For this review, take the finished solid that the model builds, in its own axes (mm). Face numbers are marked on the shaded views. A direction names the side the tool comes from. Give positions to 0.01 mm unless a question says otherwise; leave off trailing zeros. Write each loop counter-clockwise with the first axis right and the second up, starting at its lowest first coordinate (ties: lowest second). Pieces come first, ordered by that corner, then holes.
1) Wall thickness on line 1 along X through (y, z) = (-14.5, 2); line 2 along Z through (x, y) = (-6.5, -34); line 3 along X through (y, z) = (-19.25, 2.3): over which ranges is each line inside the solid? List them lowest first.
2) We need section A-A on x = 0. Give the boundary of the cut face in (y, z), and give its area (3 significant figures).
3) We need section B-B on x = 9.5. Give the boundary of the cut face in (y, z), and give its area (3 significant figures).
4) We need section C-C on x = -5.5. Give the boundary of the cut face in (y, z).
5) Machinability: for the marked faces 4 and 5, which of the approach directions +Z, -Z, +X, -X, +Y, -Y give a long, thin tool a straight path to every point of the face, cutting with its end or side? Answer none if there is none.
6) For P1, Ø2, axis at x = -5, y = -18.5, coming from the -Z side; P2, Ø1.5, axis at x = -10.5, z = -3, coming from the -Y side; P3, Ø1.5, axis at x = 8, z = -1.5, coming from the -Y side, all flat-tipped, find the tip position at first contact; note any pin that passes through.
7) Draft analysis for pull direction X (two halves, no side actions). For the marked faces 1, 2 and 3, state which applies: pulls with the +X half, pulls with the -X half, needs draft (parallel to the pull), parting line crosses it, or undercut.
from build123d import *

# Parameters (mm, degrees)
EXTRUDE_1_DEPTH     = 4
EXTRUDE_START       = -10
EXTRUDE_2_DEPTH     = 10
EXTRUDE_3_DEPTH     = 10
CUT_EXTRUDE_1_DEPTH = 80.60065996608486
FILLET_1_R          = 2


with BuildPart() as part:
    # 草图1 → 凸台-拉伸1 (new body)
    with BuildSketch(Plane.XY):
        with BuildLine():
            ThreePointArc((10.284601754984639, -12.256711089903641), (5.472322293210865, -15.035081932574474), (3.3812e-13, -16))
            Line((0, -16), (0, -17.75))
            ThreePointArc((-1.91e-15, -17.75), (1.0606601717798214, -18.189339828220177), (1.5000000000000009, -19.25))
            ThreePointArc((1.5000000000000009, -19.25), (1.0606601717798207, -20.310660171779823), (-2.94e-15, -20.75))
            Line((0, -20.75), (0, -23.100000000000005))
            ThreePointArc((-4.24e-15, -23.100000000000005), (7.900665310822955, -21.706899540154488), (14.848393783759075, -17.695626636048384))
            Line((14.848393783759088, -17.695626636048377), (10.28460175498465, -12.256711089903638))
        make_face()
        with BuildLine():
            Line((0, -17.75), (0, -16))
            ThreePointArc((3.3812e-13, -16), (-5.472322293210549, -15.035081932574588), (-10.284601754984644, -12.256711089903638))
            Line((-10.284601754984646, -12.25671108990364), (-14.848393783759084, -17.69562663604838))
            ThreePointArc((-14.848393783759082, -17.69562663604838), (-7.900665310822965, -21.706899540154485), (-4.24e-15, -23.100000000000005))
            Line((0, -23.100000000000005), (0, -20.75))
            ThreePointArc((-2.94e-15, -20.75), (-1.5000000000000009, -19.25), (-2.24e-15, -17.75))
        make_face()
    extrude(amount=EXTRUDE_1_DEPTH)

    # 草图3 → 凸台-拉伸2 (add)
    with BuildSketch(Plane.XY.offset(4).offset(EXTRUDE_START)):
        with BuildLine():
            ThreePointArc((14.848393783759091, -17.695626636048377), (3.55e-15, -23.100000000000012), (-14.848393783759086, -17.69562663604838))
            Line((-14.848393783759084, -17.69562663604838), (-17.676659266379858, -21.066222185771874))
            ThreePointArc((-17.676659266379858, -21.066222185771878), (-5.05e-15, -27.5), (17.676659266379847, -21.066222185771885))
            Line((17.67665926637986, -21.066222185771874), (14.84839378375909, -17.695626636048377))
        make_face()
    extrude(amount=EXTRUDE_2_DEPTH)

    # 草图4 → 凸台-拉伸3 (add)
    with BuildSketch(Plane.XY.offset(4).offset(EXTRUDE_START)):
        with BuildLine():
            Line((-17.67665926637985, -71.06622218577188), (17.67665926637986, -71.06622218577188))
            Line((17.67665926637986, -71.06622218577188), (17.67665926637986, -21.066222185771874))
            ThreePointArc((17.67665926637986, -21.066222185771874), (1.68e-15, -27.5), (-17.676659266379858, -21.066222185771878))
            Line((-17.676659266379858, -21.066222185771878), (-17.67665926637985, -71.06622218577188))
        make_face()
    extrude(amount=EXTRUDE_3_DEPTH)

    # 草图7 → 切除-拉伸1 (cut, through all)
    with BuildSketch(Plane(origin=(17.67665926637986, 0, 0), x_dir=(0, 0, -1), z_dir=(1, 0, 0))):
        with BuildLine():
            ThreePointArc((6, -57.06223919512314), (2.8499690271271234, -45.04655535209204), (-3.9999999999999893, -34.68425456157568))
            Line((-4, -34.68425456157568), (-4, -71.06622218577188))
            Line((-4, -71.06622218577188), (6, -71.06622218577188))
            Line((6, -71.06622218577188), (6, -57.06223919512314))
        make_face()
    extrude(amount=-CUT_EXTRUDE_1_DEPTH, mode=Mode.SUBTRACT)

    # 圆角1
    fillet_1_edges = [part.edges().sort_by_distance(p)[0] for p in [
        (10.284601754984646, -12.25671108990364, 2),
        (-10.284601754984646, -12.256711089903636, 2),
        (-14.848393783759086, -17.69562663604838, -3),
        (-17.676659266379858, -21.066222185771878, -1),
        (14.848393783759091, -17.69562663604838, -3),
        (17.676659266379858, -21.066222185771885, -1),
        (17.67665926637986, -45.04655535209205, -2.8499690271271234),
        (3.55e-15, -34.68425456157568, 3.999999999999993),
        (3.55e-15, -57.06223919512314, -6),
        (-17.676659266379854, -45.04655535209205, -2.8499690271271234),
    ]]
    fillet(fillet_1_edges, radius=FILLET_1_R)


solid = part.part
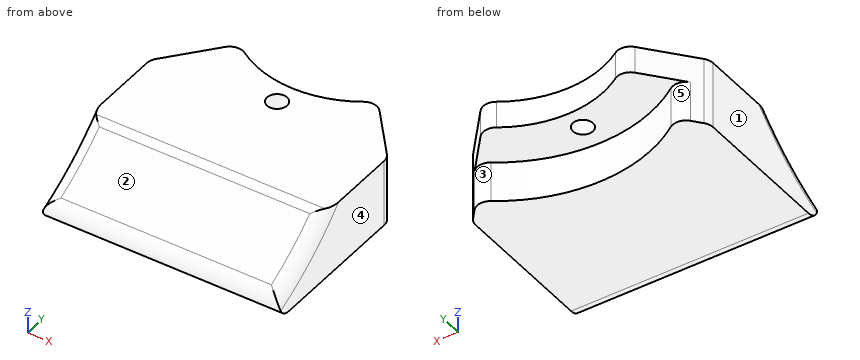
Results list:
1. line 1: x = -12.17 to -6.76, 6.76 to 12.17
1. line 2: z = -6 to 4
1. line 3: x = -16.15 to -1.5, 1.5 to 16.15
2. outline: (-43.68, -2.21) arc R2 ccw to (-42.79, -6) - (-23.1, -6) - (-23.1, 0) - (-20.75, 0) - (-20.75, 4) - (-33.91, 4) arc R2 ccw to (-35.24, 3.49) arc R38.07 cw to start; (-17.75, 0) - (-16, 0) - (-16, 4) - (-17.75, 4) - close
2. area: 194 mm2
3. outline: (-43.68, -2.21) arc R2 ccw to (-42.79, -6) - (-21.06, -6) - (-21.06, 0) - (-13.04, 0) - (-13.04, 4) - (-33.91, 4) arc R2 ccw to (-35.24, 3.49) arc R38.07 cw to start
3. area: 230 mm2
4. outline: (-43.68, -2.21) arc R2 ccw to (-42.79, -6) - (-22.44, -6) - (-22.44, 0) - (-15.02, 0) - (-15.02, 4) - (-33.91, 4) arc R2 ccw to (-35.24, 3.49) arc R38.07 cw to start
5. face 4: +Z, -Z, +X, +Y, -Y
5. face 5: -Z, +Y
6. P1: stops at z = 0
6. P2: stops at y = -44.78
6. P3: stops at y = -43.76
7. face 1: pulls with the -X half
7. face 2: needs draft
7. face 3: undercut
